For this review, use the dimensioned drawing (mm, ordinates from the lowest corner) and the shaded views. A direction names the side the tool comes from. Coordinates: 2 decimals unless noted, no trailing zeros. Write each loop counter-clockwise with the first axis right and the second up, starting at its lowest first coordinate (ties: lowest second). Pieces come first, ordered by that corner, then holes.
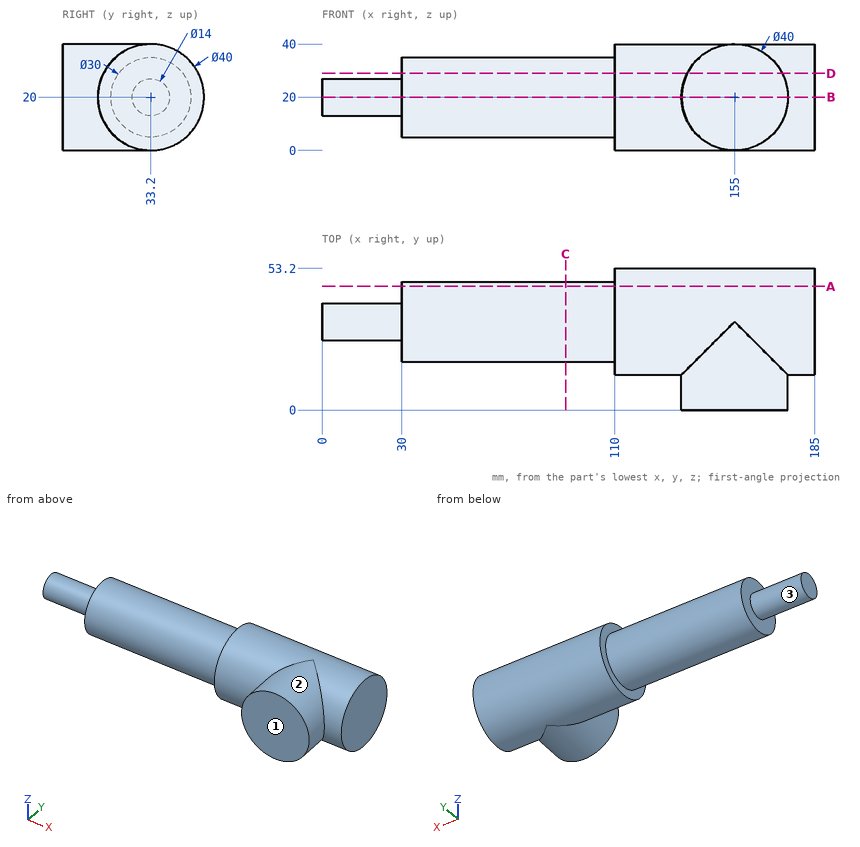
(1) Consider section B-B (z = 20). Give the boundary of the cut face in (x, y).
(2) Wall thickness on line 1 (X direction, y = 25, z = 20); line 2 (X direction, y = 40.5, z = 6); line 3 (Y direction, x = 8, z = 21.5): over which ranges is each line inside the solid? List them lowest first.
(3) Insertion check: pin 1 Ø12 at (x, z) = (37.5, 20.5) entering from +Y; pin 2 Ø8 at (x, z) = (100.5, 14.5) entering from -Y; pin 3 Ø5 at (x, y) = (124.5, 22.5) entering from +Z. Each pin has a flat end and moves straight along its axis. Give the tip position at first contact, or say it passes through.
(4) For the marked faces 1, 2 and 3, list the 3-axis set-ups (+Z, -Z, +X, -X, +Y, -Y) from which the entire face can be reached by the end or side of a thin tool; tool diameter is ignored.
(5) Consider section C-C (x = 91.5). Give the boundary of the cut face in (y, z).
(6) Consider section A-A (y = 46.5). Give the boundary of the cut face in (x, z).
(7) Consider section D-D (z = 29). Give the boundary of the cut face in (x, y).
Results:
1. outline: (0, 26.2) - (30, 26.2) - (30, 18.2) - (110, 18.2) - (110, 13.2) - (135, 13.2) - (135, 0) - (175, 0) - (175, 13.2) - (185, 13.2) - (185, 53.2) - (110, 53.2) - (110, 48.2) - (30, 48.2) - (30, 40.2) - (0, 40.2) - close
2. line 1: x = 30 to 185
2. line 2: x = 110 to 185
2. line 3: y = 26.36 to 40.04
3. pin 1: stops at y = 48.2
3. pin 2: stops at y = 18.28
3. pin 3: stops at z = 38.24
4. face 1: +Z, -Z, +X, -X, -Y
4. face 2: -Y
4. face 3: -X
5. outline: circle Ø30 at (33.2, 20)
6. outline: (30, 13.06) - (110, 13.06) - (110, 5.06) - (185, 5.06) - (185, 34.94) - (110, 34.94) - (110, 26.94) - (30, 26.94) - close
7. outline: (30, 21.2) - (110, 21.2) - (110, 15.34) - (137.14, 15.34) - (137.14, 0) - (172.86, 0) - (172.86, 15.34) - (185, 15.34) - (185, 51.06) - (110, 51.06) - (110, 45.2) - (30, 45.2) - close
